from build123d import *

# Parameters (mm, degrees)
F1_DEPTH       = 42.5
F2_C1_SIZE2    = 0.3
F2_C1_SIZE     = 0.388
F2_C2_SIZE2    = 0.388
F2_C2_SIZE     = 0.3
F3_SIZE        = 0.4
F5_D           = 2.4
F5_CBORE_D     = 4.2
F5_CBORE_DEPTH = 2.3


with BuildPart() as f1:
    # F0 (on Front) → F1 (new body, symmetric)
    with BuildSketch(Plane.XZ):
        with BuildLine():
            Line((-3.5, 0), (3.5, 0))
            Line((3.5, 0), (3.5, 2.3493352987))
            ThreePointArc((3.5, 2.3493352987), (3.4856956825, 2.4008741191), (3.446875, 2.4376683864))
            ThreePointArc((3.446875, 2.4376683864), (3.2976460443, 2.5440105461), (3.1811284368, 2.6854375))
            ThreePointArc((3.1811284368, 2.6854375), (3.1447986618, 2.7199464122), (3.096289642, 2.7325))
            Line((3.096289642, 2.7325), (2.7685954715, 2.7325))
            ThreePointArc((2.7685954715, 2.7325), (2.285, 3.056), (2.7685954715, 3.3795))
            Line((2.7685954715, 3.3795), (3.096289642, 3.3795))
            ThreePointArc((3.096289642, 3.3795), (3.1447986618, 3.3920535878), (3.1811284368, 3.4265625))
            ThreePointArc((3.1811284368, 3.4265625), (3.2976460443, 3.5679894539), (3.446875, 3.6743316136))
            ThreePointArc((3.446875, 3.6743316136), (3.4856956825, 3.7111258809), (3.5, 3.7626647013))
            Line((3.5, 3.7626647013), (3.5, 4.8))
            Line((3.5, 4.8), (-3.5, 4.8))
            Line((-3.5, 4.8), (-3.5, 3.7626647013))
            ThreePointArc((-3.5, 3.7626647013), (-3.4856956825, 3.7111258809), (-3.446875, 3.6743316136))
            ThreePointArc((-3.446875, 3.6743316136), (-3.2976460443, 3.5679894539), (-3.1811284368, 3.4265625))
            ThreePointArc((-3.1811284368, 3.4265625), (-3.1447986618, 3.3920535878), (-3.096289642, 3.3795))
            Line((-3.096289642, 3.3795), (-2.7685954715, 3.3795))
            ThreePointArc((-2.7685954715, 3.3795), (-2.4403958056, 3.3469109959), (-2.285, 3.056))
            ThreePointArc((-2.285, 3.056), (-2.4403958056, 2.7650890041), (-2.7685954715, 2.7325))
            Line((-2.7685954715, 2.7325), (-3.096289642, 2.7325))
            ThreePointArc((-3.096289642, 2.7325), (-3.1447986618, 2.7199464122), (-3.1811284368, 2.6854375))
            ThreePointArc((-3.1811284368, 2.6854375), (-3.2976460443, 2.5440105461), (-3.446875, 2.4376683864))
            ThreePointArc((-3.446875, 2.4376683864), (-3.4856956825, 2.4008741191), (-3.5, 2.3493352987))
            Line((-3.5, 2.3493352987), (-3.5, 0))
        make_face()
    extrude(amount=F1_DEPTH, both=True)

    # F2: chamfer of 0.3 x 0.388 on 2 edges, made by hand

    # F2_c1
    f2_c1_edges = [f1.edges().sort_by_distance(p)[0] for p in [
        (-3.5, 0, 4.8),
    ]]
    f2_c1_side = f1.faces().sort_by_distance((-3.5, 0, 4.794))[0]
    chamfer(f2_c1_edges, length=F2_C1_SIZE, length2=F2_C1_SIZE2, reference=f2_c1_side)

    # F2_c2
    f2_c2_edges = [f1.edges().sort_by_distance(p)[0] for p in [
        (3.5, 0, 4.8),
    ]]
    f2_c2_side = f1.faces().sort_by_distance((3.494, 0, 4.8))[0]
    chamfer(f2_c2_edges, length=F2_C2_SIZE, length2=F2_C2_SIZE2, reference=f2_c2_side)

    # F3
    f3_edges = [f1.edges().sort_by_distance(p)[0] for p in [
        (3.5, 0, 0),
        (-3.5, 0, 0),
    ]]
    chamfer(f3_edges, length=F3_SIZE)

    # F5 (through all)
    with Locations(Plane.XY.offset(4.8)):
        with Locations((0, 30), (0, 15), (0, 0), (0, -15), (0, -30)):
            CounterBoreHole(F5_D / 2, F5_CBORE_D / 2, F5_CBORE_DEPTH)


solid = f1.part
Read the model definition and answer for the solid it produces. Units are mm, in the model's axes. A direction names the side the tool comes from. Give positions to 0.01 mm unless a question says otherwise; leave off trailing zeros. Write each loop counter-clockwise with the first axis right and the second up, starting at its lowest first coordinate (ties: lowest second). Pieces come first, ordered by that corner, then holes. Notation, with made-up numbers: (-31.75, -10) - (11.25, -10) arc R7 cw to (11.25, 3) - close; hole circle Ø6 at (-39.75, 39). An arc over 180 degrees is marked (long way). Use CSV: the item, a comma, the result in double quotes. Start each with the question number.
(1) Determine the mould class of faces 1 (the flat face through (0, -42.5, 2)), 2 (the flat face through (-3.5, -1, 1)), 3 (the flat face through (1, -31, 2.5)), 4 (the flat face through (3.5, -1, 1)) for opening direction X: +X half, -X half, draft (parallel to the pull), parting line (faces both ways), or undercut.
(2) Consider line 1 along Y through (x, z) = (0, 3.9); line 2 along Z through (x, y) = (-3, 38); line 3 along Y through (x, z) = (0, 1.95). Determine where each line is inside the solid, lowest interval first.
(3) Find section A-A (z = 1.1). Give the vertices of the cut face in (x, y), plus the area to 3 significant figures.
(4) For faces 5 (the cylindrical face through (-0.273, -12.918, 3.666)), 6 (the cylindrical face through (0.26, 13.83, 1.23)), determine the directions among +Z, -Z, +X, -X, +Y, -Y from which every point of the face is accessible in a straight line to the end or side of a thin tool.
(5) Given P1, Ø1.9, axis at x = 0, y = 0, coming from the +Z side; P2, Ø3.5, axis at x = 0, y = 30, coming from the +Z side, each flat-ended and moving along its own axis, determine where each tip first touches the part or whether it passes through.
(6) Find section C-C (x = 0). Count the separate pieces of the cut face and the enclosed holes in it, plus the area to 3 significant figures.
Findings below:
1,face 1,"draft"
1,face 2,"-X half"
1,face 3,"undercut"
1,face 4,"+X half"
2,line 1,"-42.5 to -32.1, -27.9 to -17.1, -12.9 to -2.1, 2.1 to 12.9, 17.1 to 27.9, 32.1 to 42.5"
2,line 2,"0 to 2.73, 3.38 to 4.8"
2,line 3,"-42.5 to -31.2, -28.8 to -16.2, -13.8 to -1.2, 1.2 to 13.8, 16.2 to 28.8, 31.2 to 42.5"
3,outline,"(-3.5, -42.5) - (3.5, -42.5) - (3.5, 42.5) - (-3.5, 42.5) - close; hole circle Ø2.4 at (0, -30); hole circle Ø2.4 at (0, -15); hole circle Ø2.4 at (0, 0); hole circle Ø2.4 at (0, 15); hole circle Ø2.4 at (0, 30)"
3,area,"572 mm2"
4,face 5,"+Z"
4,face 6,"+Z, -Z"
5,P1,"through"
5,P2,"z = 2.5"
6,separate pieces,"6"
6,enclosed holes,"0"
6,area,"330 mm2"
